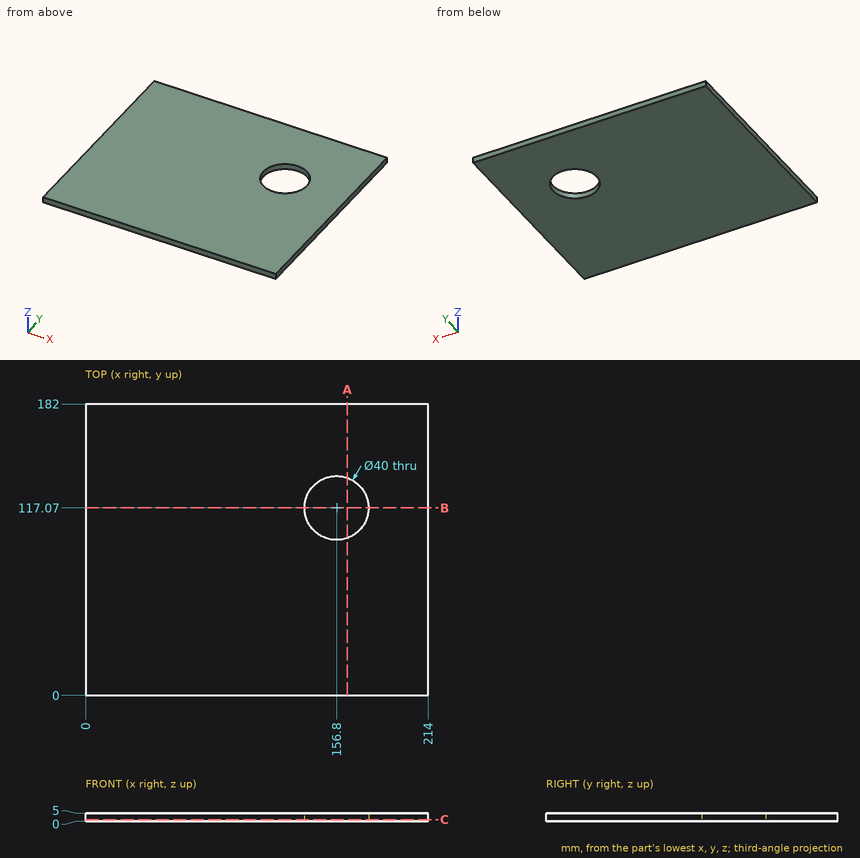
Geometry check sheet. Reference: drawing and pictorial views, mm from the part's lowest x, y, z. Give positions to 0.01 mm unless a question says otherwise; leave off trailing zeros. Order: outer loops, then holes, each group sorted by start corner. A loop starts at its lowest first (then second) coordinate and runs counter-clockwise, first axis right, second up. Notation, with made-up numbers: M 7.25,-17 L 27.25,-17 A17 ccw 27.25,-3 Z; hole C 57,4.5 d10. An arc over 180 degrees is marked long. Answer as a JSON object with one key per item and string values. Group by question number.
1) Cross-section at B-B (y = 117.07). Enter the section's corners in (x, z).
2) Cross-section at A-A (x = 163.5). Enter the section's corners in (y, z), then the cut area to 3 significant figures.
3) Scan lines: line 1 along Y through (x, z) = (156.8, 3.05); line 2 along X through (y, z) = (100.5, 3.5); line 3 along X through (y, z) = (99.5, 4.1). Record each from-to range of solid material in increasing order. Write a range as [from, to].
4) Cross-section at C-C (z = 1.1). Enter the section's corners in (x, y).
Result sheet:
{
 "1": {"outline": "M 0,0 L 136.8,0 L 136.8,5 L 0,5 Z; M 176.8,0 L 214,0 L 214,5 L 176.8,5 Z"},
 "2": {"outline": "M 0,0 L 98.23,0 L 98.23,5 L 0,5 Z; M 135.91,0 L 182,0 L 182,5 L 135.91,5 Z", "area": "722 mm2"},
 "3": {"line 1": "y = [0, 97.07], [137.07, 182]", "line 2": "x = [0, 145.6], [168, 214]", "line 3": "x = [0, 147.25], [166.35, 214]"},
 "4": {"outline": "M 0,0 L 214,0 L 214,182 L 0,182 Z; hole C 156.8,117.07 d40"}
}
